from build123d import *

# Parameters (mm, degrees)
F1_R     = 2
F2_DEPTH = 12
F3_R     = 1
F4_R     = 0.2
F5_R     = 1.25
F6_DEPTH = 10


with BuildPart() as f2:
    # F1 (on Front) → F2 (new body)
    with BuildSketch(Plane.XZ):
        Circle(F1_R)
    extrude(amount=F2_DEPTH)

    # F3
    f3_edges = [f2.edges().sort_by_distance(p)[0] for p in [
        (-2, -12, 0),
    ]]
    fillet(f3_edges, radius=F3_R)

    # F4
    f4_edges = [f2.edges().sort_by_distance(p)[0] for p in [
        (-2, 0, 0),
    ]]
    fillet(f4_edges, radius=F4_R)

    # F5 (on face) → F6 (cut)
    with BuildSketch(Plane(origin=(0, 0, 0), x_dir=(-1, 0, 0), z_dir=(0, 1, 0))):
        Circle(F5_R)
    extrude(amount=-F6_DEPTH, mode=Mode.SUBTRACT)


solid = f2.part
Geometry: final body of the model. Coordinates: model frame, mm. A direction names the side the tool comes from. Give positions to 0.01 mm unless a question says otherwise; leave off trailing zeros. Order: outer loops, then holes, each group sorted by start corner. A loop starts at its lowest first (then second) coordinate and runs counter-clockwise, first axis right, second up. Notation, with made-up numbers: (51.25, -35) - (66.25, -35) arc R26 ccw to (66.25, -19) - close; hole circle Ø8 at (21.25, 34.5). An arc over 180 degrees is marked (long way). Use CSV: the item, a comma, the result in double quotes.
1. Material intervals for line 1 along Z through (x, y) = (0, -5); line 2 along Y through (x, z) = (0.9, -0.15); line 3 along X through (y, z) = (-9, -0.7), sorted ascending. Write a range as from..to.
Answers below:
line 1,"-2..-1.25, 1.25..2"
line 2,"-12..-10"
line 3,"-1.87..-1.04, 1.04..1.87"
2. Access query for faces 4 (the face through (0, -12, 0)), 5 (the face through (0.27, -4.93, -1.22)). Directions: +Z, -Z, +X, -X, +Y, -Y. A direction counts if a zero-diameter tool reaches every point of the face in a straight line with its end or side. Return the directions, or none.
Answers below:
face 4,"+Z, -Z, +X, -X, -Y"
face 5,"+Y"
3. Section query A-A (y = -5.75). Output: boundary loops of the cut face in (x, z).
Answers below:
outline,"circle Ø4 at (0, 0); hole circle Ø2.5 at (0, 0)"
4. Mould query, pull axis X, two halves, no side actions, for faces 1 (the face through (1, 0, -1)), 2 (the face through (0, -6, -2)), 3 (the face through (0, -10, 0)). Classes: +X half, -X half, draft (parallel to the pull), parting line (faces both ways), or undercut.
Answers below:
face 1,"draft"
face 2,"parting line"
face 3,"undercut"
5. Contact query for a flat-ended pin moving along its axis: pin 1 (1.5 mm diameter, centred on x = -1.5, y = -4, fed in from -Z). Output: stop coordinate, or through.
Answers below:
pin 1,"z = -1.85"
